Build history of the part. All positions in model axes, mm. Round coordinates to 2 decimals unless told otherwise and drop trailing zeros. Order: outer loops, then holes, each group sorted by start corner. A loop starts at its lowest first (then second) coordinate and runs counter-clockwise, first axis right, second up. Notation, with made-up numbers: (22.25, 64.25) -> (29.25, 64.25) arc R19 ccw to (29.25, 68.25) -> close; hole circle Ø11 at (19.5, -15). An arc over 180 degrees is marked (long way). Use a Markdown table: item, result. Add a question column.
Item 1: Slice it at A-A, the plane z = -39.5. Give the cut face in (x, y).
Item 2: Slice it at B-B, the plane y = 451. Give the cut face in (x, z) (3 decimals), plus the area to 3 significant figures.
Item 3: Pin check, flat tips, straight feed: pin 1 (4 mm diameter, centred on x = 21.5, y = 24.5, fed in from -Z); pin 2 (4.5 mm diameter, centred on y = -78.62, z = -28.58, fed in from +X). Stop position of each tip, or through.
Item 4: Probe L1, parallel to X at y = 278.5, z = -10; L2, parallel to Z at x = 5.5, y = 471; L3, parallel to Z at x = 34, y = 76.5. List the from-to ranges inside material, lowest first.
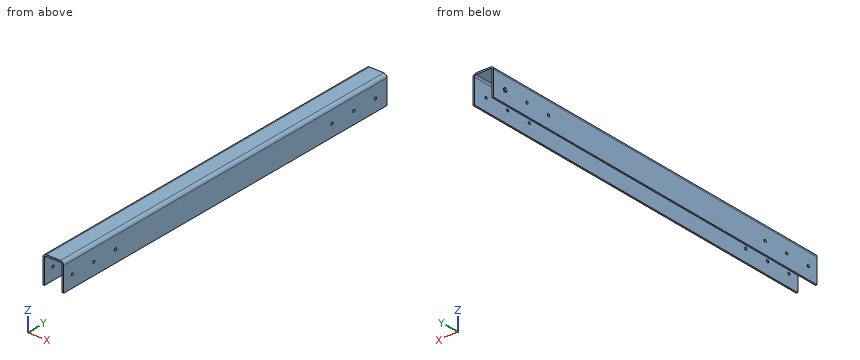
from build123d import *

# Parameters (mm, degrees)
SKETCH1_W                            = 38.1
SKETCH1_H                            = 749.3
BASE_FLANGE1_DEPTH                   = 2.65684
EDGE_FLANGE1_STRIP_W                 = 16.97736
EDGE_FLANGE1_STRIP_H                 = 2.65684
EDGE_FLANGE1_STRIP_CUT_DEPTH         = 749.3
EDGE_FLANGE1_STRIP_2_W               = 16.97736
EDGE_FLANGE1_STRIP_2_H               = 2.65684
EDGE_FLANGE1_STRIP_CUT_2_DEPTH       = 749.3
EDGE_FLANGE1_DEPTH                   = 749.3
EDGE_FLANGE1_BEND_DEPTH              = 749.3
CUT_EXTRUDE1_START                   = -38.1
CUT_EXTRUDE1_OUTLINE_W               = 50.8
CUT_EXTRUDE1_OUTLINE_H               = 38.1
CUT_EXTRUDE1_DEPTH                   = 38.1
F_10_0_1935_DIAMETER_HOLE1_D         = 4.9149
F_19_64_0_29688_DIAMETER_HOLE3_D     = 7.540752
F_19_64_0_29688_DIAMETER_HOLE3_DEPTH = 35.44216


# Read off the part's stored shape, not the designer's step: Cut-Extrude1
# Sheet-metal steps are written as plain solids
with BuildPart() as part:
    # Sketch1 → Base-Flange1 (new body)
    with BuildSketch(Plane.XY):
        with Locations((19.05, 276.978929766)):
            Rectangle(SKETCH1_W, SKETCH1_H)
    extrude(amount=-BASE_FLANGE1_DEPTH)

    # Edge-Flange1 strip (across the edge) → Edge-Flange1 strip cut (cut)
    with BuildSketch(Plane(origin=(38.1, 651.628929766, -2.65684), x_dir=(-1, 0, 0), z_dir=(0, -1, 0))):
        with Locations((-2.65684, -1.32842)):
            Rectangle(EDGE_FLANGE1_STRIP_W, EDGE_FLANGE1_STRIP_H)
    extrude(amount=EDGE_FLANGE1_STRIP_CUT_DEPTH, mode=Mode.SUBTRACT)

    # Edge-Flange1 strip 2 (across the edge) → Edge-Flange1 strip cut 2 (cut)
    with BuildSketch(Plane(origin=(0, -97.671070234, -2.65684), x_dir=(1, 0, 0), z_dir=(0, 1, 0))):
        with Locations((-2.65684, -1.32842)):
            Rectangle(EDGE_FLANGE1_STRIP_2_W, EDGE_FLANGE1_STRIP_2_H)
    extrude(amount=EDGE_FLANGE1_STRIP_CUT_2_DEPTH, mode=Mode.SUBTRACT)

    # Edge-Flange1 section (across the edge) → Edge-Flange1 (add)
    with BuildSketch(Plane(origin=(38.1, 651.628929766, -2.65684), x_dir=(-1, 0, 0), z_dir=(0, -1, 0))):
        with BuildLine():
            Line((0, 3.175), (0, 48.14316))
            Line((0, 48.14316), (2.65684, 48.14316))
            Line((2.65684, 48.14316), (2.65684, 3.175))
            ThreePointArc((2.65684, 3.175), (3.58677597, 0.92993597), (5.83184, 0))
            Line((5.83184, 0), (5.83184, -2.65684))
            ThreePointArc((5.83184, -2.65684), (1.708106389, -0.948733611), (0, 3.175))
        make_face()
    extrude(amount=EDGE_FLANGE1_DEPTH)

    # Edge-Flange1 section 2 (across the edge) → Edge-Flange1 bend (add)
    with BuildSketch(Plane(origin=(0, -97.671070234, -2.65684), x_dir=(1, 0, 0), z_dir=(0, 1, 0))):
        with BuildLine():
            Line((0, 3.175), (0, 48.14316))
            Line((0, 48.14316), (2.65684, 48.14316))
            Line((2.65684, 48.14316), (2.65684, 3.175))
            ThreePointArc((2.65684, 3.175), (3.58677597, 0.92993597), (5.83184, 0))
            Line((5.83184, 0), (5.83184, -2.65684))
            ThreePointArc((5.83184, -2.65684), (1.708106389, -0.948733611), (0, 3.175))
        make_face()
    extrude(amount=EDGE_FLANGE1_BEND_DEPTH)

    # Cut-Extrude1 outline → Cut-Extrude1 (cut)
    with BuildSketch(Plane(origin=(38.1, 0, 0), x_dir=(0, 0, -1), z_dir=(1, 0, 0)).offset(CUT_EXTRUDE1_START)):
        with Locations((25.4, 632.578929766)):
            Rectangle(CUT_EXTRUDE1_OUTLINE_W, CUT_EXTRUDE1_OUTLINE_H)
    extrude(amount=CUT_EXTRUDE1_DEPTH, mode=Mode.SUBTRACT)

    # #10 (0.1935) Diameter Hole1 (through all)
    with Locations(Plane(origin=(38.1, 0, 0), x_dir=(0, 0, -1), z_dir=(1, 0, 0))):
        with Locations((28.575, -78.621070234), (28.575, -30.996070234), (28.575, 16.628929766), (28.575, 588.128929766), (28.575, 540.503929766), (28.575, 492.878929766)):
            Hole(F_10_0_1935_DIAMETER_HOLE1_D / 2)

    # 19/64 (0.29688) Diameter Hole3
    with Locations(Plane.ZY):
        with Locations((-28.575, 588.128929766)):
            Hole(F_19_64_0_29688_DIAMETER_HOLE3_D / 2, depth=F_19_64_0_29688_DIAMETER_HOLE3_DEPTH)


solid = part.part
Check sheet entries:
| question | item | result |
|---|---|---|
| 1 | outline | (0, -97.67) -> (2.66, -97.67) -> (2.66, 613.53) -> (0, 613.53) -> close; (35.44, -97.67) -> (38.1, -97.67) -> (38.1, 613.53) -> (35.44, 613.53) -> close |
| 2 | outline | (0, -50.8) -> (2.657, -50.8) -> (2.657, -5.832) arc R3.175 cw to (5.832, -2.657) -> (32.268, -2.657) arc R3.175 cw to (35.443, -5.832) -> (35.443, -50.8) -> (38.1, -50.8) -> (38.1, -5.832) arc R5.832 ccw to (32.268, 0) -> (5.832, 0) arc R5.832 ccw to (0, -5.832) -> close |
| 2 | area | 347 mm2 |
| 3 | pin 1 | z = -2.66 |
| 3 | pin 2 | through |
| 4 | L1 | 0 to 2.66, 35.44 to 38.1 |
| 4 | L2 | -2.67 to -0.01 |
| 4 | L3 | -3.17 to -0.26 |
